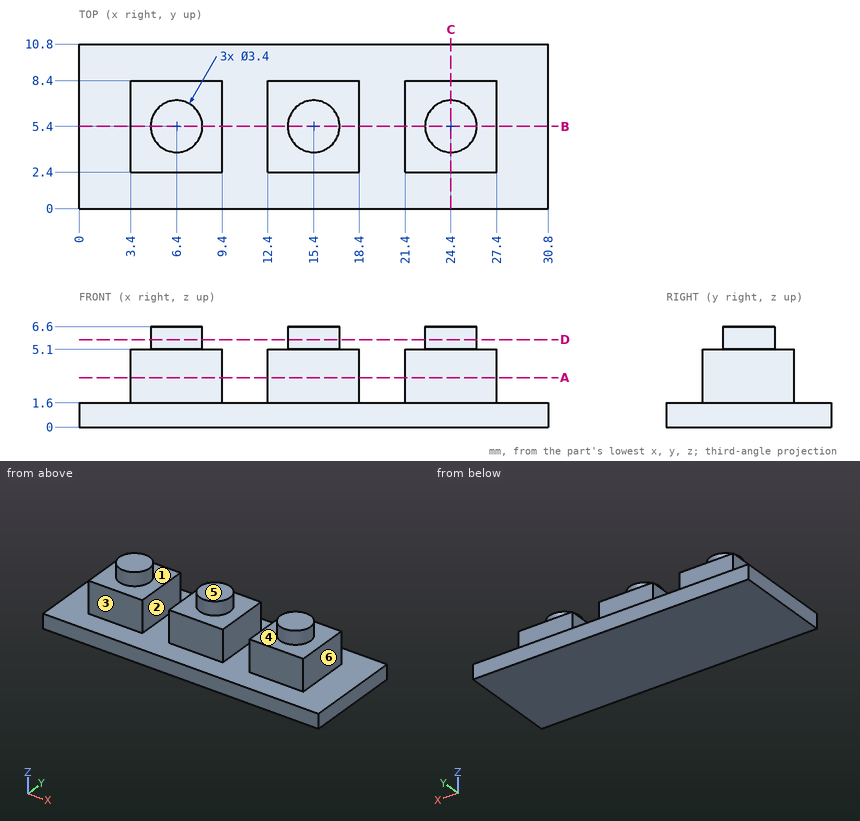
Drawing for the job (mm, zero at the part's lowest x, y, z). A direction names the side the tool comes from. Round coordinates to 2 decimals unless told otherwise and drop trailing zeros. Write each loop counter-clockwise with the first axis right and the second up, starting at its lowest first coordinate (ties: lowest second). Pieces come first, ordered by that corner, then holes. Notation, with made-up numbers: M -12,49 L 0,49 A24 cw 0,66 Z; hole C -2.75,62.25 d4. An arc over 180 degrees is marked long. Answer in a Markdown table with one row per item.
1. Saw through at C-C (x = 24.4). List the corners of the cut face in (y, z).
Geometry check:
| item | result |
|---|---|
| outline | M 0,0 L 10.8,0 L 10.8,1.6 L 8.4,1.6 L 8.4,5.1 L 7.1,5.1 L 7.1,6.6 L 3.7,6.6 L 3.7,5.1 L 2.4,5.1 L 2.4,1.6 L 0,1.6 Z |
2. Probe L1, parallel to X at y = 7, z = 3.5; L2, parallel to Z at x = 19.5, y = 6.75; L3, parallel to Z at x = 3.5, y = 7. List the from-to ranges inside material, lowest first. Write a range as [from, to].
Geometry check:
| item | result |
|---|---|
| L1 | [3.4, 9.4], [12.4, 18.4], [21.4, 27.4] |
| L2 | [0, 1.6] |
| L3 | [0, 5.1] |
3. Saw through at B-B (y = 5.4). List the corners of the cut face in (x, z).
Geometry check:
| item | result |
|---|---|
| outline | M 0,0 L 30.8,0 L 30.8,1.6 L 27.4,1.6 L 27.4,5.1 L 26.1,5.1 L 26.1,6.6 L 22.7,6.6 L 22.7,5.1 L 21.4,5.1 L 21.4,1.6 L 18.4,1.6 L 18.4,5.1 L 17.1,5.1 L 17.1,6.6 L 13.7,6.6 L 13.7,5.1 L 12.4,5.1 L 12.4,1.6 L 9.4,1.6 L 9.4,5.1 L 8.1,5.1 L 8.1,6.6 L 4.7,6.6 L 4.7,5.1 L 3.4,5.1 L 3.4,1.6 L 0,1.6 Z |
4. Mould opens along X. For the marked faces 4, 5 and 6 say: +X half, -X half, draft (parallel to the pull), parting line (faces both ways), or undercut.
Geometry check:
| item | result |
|---|---|
| face 4 | undercut |
| face 5 | draft |
| face 6 | +X half |
5. Which spindle directions (+Z, -Z, +X, -X, +Y, -Y) get a long thin tool onto all of the face, cutting with end or side? Do the marked faces 1, 2 and 3. Say none if no direction does.
Geometry check:
| item | result |
|---|---|
| face 1 | +Z |
| face 2 | +Z, +Y, -Y |
| face 3 | +Z, +X, -X, -Y |
6. Saw through at D-D (z = 5.75). List the corners of the cut face in (x, y), and give its area (3 significant figures).
Geometry check:
| item | result |
|---|---|
| outline | C 6.4,5.4 d3.4; C 15.4,5.4 d3.4; C 24.4,5.4 d3.4 |
| area | 27.2 mm2 |
7. Flat gauge pins, fed straight in: P1, Ø1, axis at x = 6, z = 2.5, coming from the +Y side; P2, Ø1, axis at x = 23.5, z = 2.5, coming from the -Y side; P3, Ø1.7, axis at y = 4, z = 3.5, coming from the +X side. Where does each tip first touch, or does it go through?
Geometry check:
| item | result |
|---|---|
| P1 | y = 8.4 |
| P2 | y = 2.4 |
| P3 | x = 27.4 |
8. Saw through at A-A (z = 3.25). List the corners of the cut face in (x, y).
Geometry check:
| item | result |
|---|---|
| outline | M 3.4,2.4 L 9.4,2.4 L 9.4,8.4 L 3.4,8.4 Z; M 12.4,2.4 L 18.4,2.4 L 18.4,8.4 L 12.4,8.4 Z; M 21.4,2.4 L 27.4,2.4 L 27.4,8.4 L 21.4,8.4 Z |
